Source: three-view drawing plus pictorial views. Frame: mm from the lowest corner of the part. Round coordinates to 2 decimals unless told otherwise and drop trailing zeros. Order: outer loops, then holes, each group sorted by start corner. A loop starts at its lowest first (then second) coordinate and runs counter-clockwise, first axis right, second up. Notation, with made-up numbers: (3.25, -32) -> (24.25, -32) arc R15 cw to (24.25, -23) -> close; hole circle Ø1 at (-28.5, 89.25). An arc over 180 degrees is marked (long way). Answer as CSV lines item,"result".
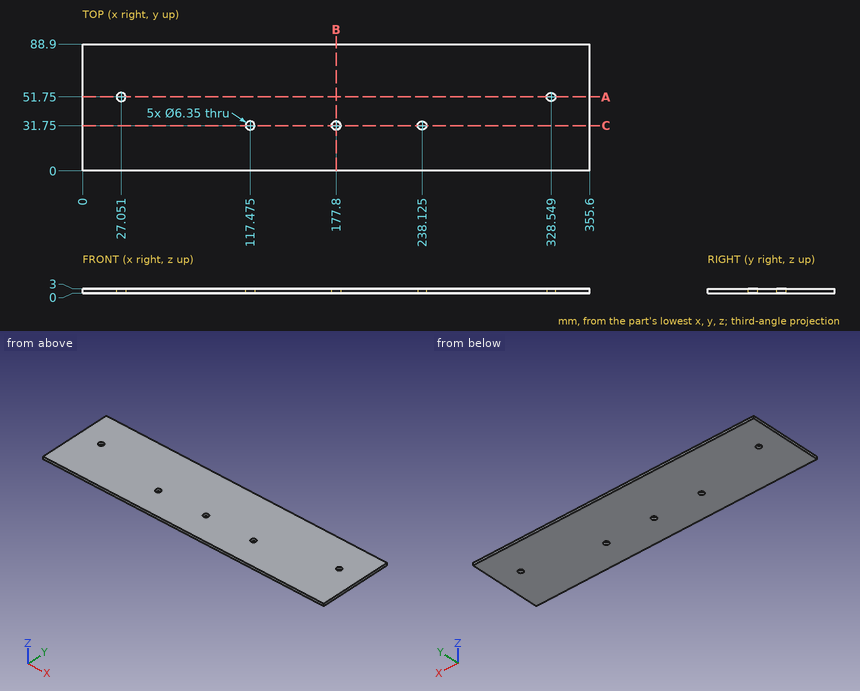
1. Section query C-C on y = 31.75. Return loops of the section in (x, z) (3 decimals), and give its area (3 significant figures).
Results below:
outline,"(0, 0) -> (114.3, 0) -> (114.3, 3) -> (0, 3) -> close; (120.65, 0) -> (174.625, 0) -> (174.625, 3) -> (120.65, 3) -> close; (180.975, 0) -> (234.95, 0) -> (234.95, 3) -> (180.975, 3) -> close; (241.3, 0) -> (355.6, 0) -> (355.6, 3) -> (241.3, 3) -> close"
area,"1,010 mm2"
2. Line query: L1, parallel to Y at x = 177.8, z = 1.1 (3 decimals); L2, parallel to X at y = 54, z = 0.3. Output: solid intervals per line, ascending. Write a range as [from, to].
Results below:
L1,"[0, 28.575], [34.925, 88.9]"
L2,"[0, 24.81], [29.29, 326.31], [330.79, 355.6]"
3. Section query A-A on y = 51.75. Return loops of the section in (x, z), and give its area (3 significant figures).
Results below:
outline,"(0, 0) -> (23.88, 0) -> (23.88, 3) -> (0, 3) -> close; (30.23, 0) -> (325.37, 0) -> (325.37, 3) -> (30.23, 3) -> close; (331.72, 0) -> (355.6, 0) -> (355.6, 3) -> (331.72, 3) -> close"
area,"1,030 mm2"
4. Section query B-B on x = 177.8. Return loops of the section in (y, z) (3 decimals), and give its area (3 significant figures).
Results below:
outline,"(0, 0) -> (28.575, 0) -> (28.575, 3) -> (0, 3) -> close; (34.925, 0) -> (88.9, 0) -> (88.9, 3) -> (34.925, 3) -> close"
area,"248 mm2"
